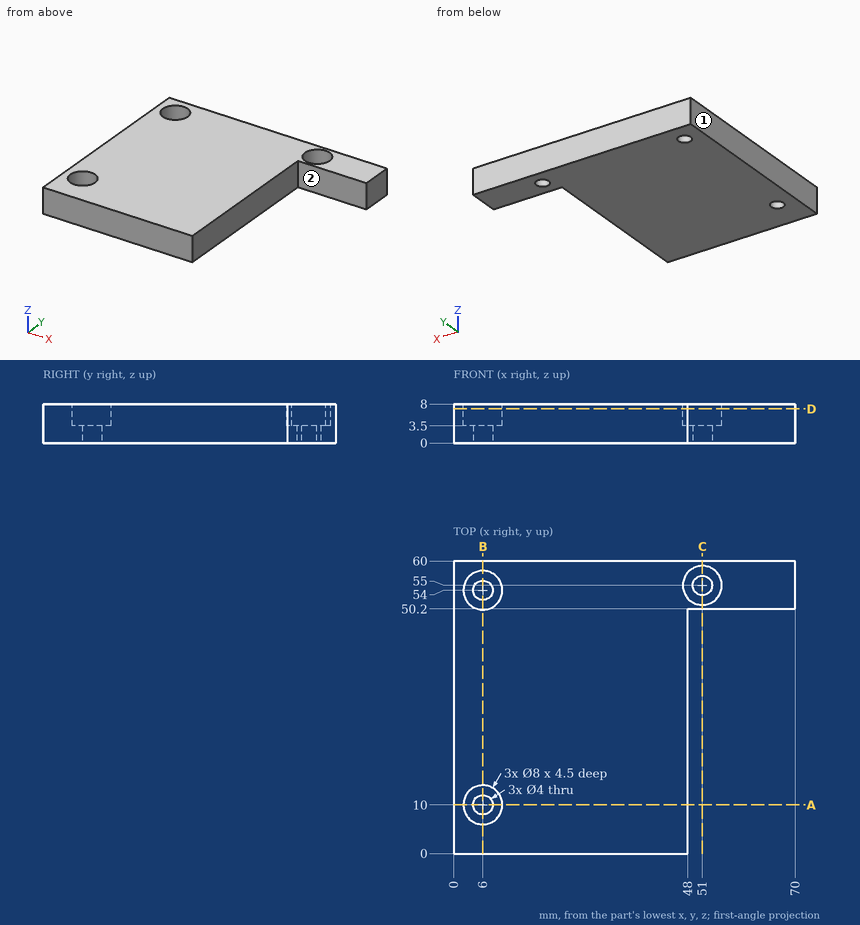
Part print with two shaded views. Sizes in mm from the minimum x, y, z corner. A direction names the side the tool comes from. Round coordinates to 2 decimals unless told otherwise and drop trailing zeros. Order: outer loops, then holes, each group sorted by start corner. A loop starts at its lowest first (then second) coordinate and runs counter-clockwise, first axis right, second up. Notation, with made-up numbers: (25, -27.5) - (29, -27.5) arc R23 cw to (29, 8.5) - close; hole circle Ø3 at (-28.75, 25). An arc over 180 degrees is marked (long way). Return JSON: item names as keys, results as strings.
(1) Wall check: probe 1 along Y at (x, z) = (6, 4.9); probe 2 along Y at (x, z) = (6, 2.5); probe 3 along Y at (x, z) = (59.5, 4.75). Give the ranges that are in metal, low to high. Write a range as from..to.
Answer key:
{"probe 1": "y = 0..6, 14..50, 58..60", "probe 2": "y = 0..8, 12..52, 56..60", "probe 3": "y = 50.2..60"}
(2) Cut at A-A (y = 10). Give the cut face in (x, z), then the cut area to 3 significant figures.
Answer key:
{"outline": "(0, 0) - (4, 0) - (4, 3.5) - (2, 3.5) - (2, 8) - (0, 8) - close; (8, 0) - (48, 0) - (48, 8) - (10, 8) - (10, 3.5) - (8, 3.5) - close", "area": "334 mm^2"}
(3) Cut at D-D (z = 7). Give the cut face in (x, y), then the cut area to 3 significant figures.
Answer key:
{"outline": "(0, 0) - (48, 0) - (48, 50.2) - (70, 50.2) - (70, 60) - (0, 60) - close; hole circle Ø8 at (6, 10); hole circle Ø8 at (6, 54); hole circle Ø8 at (51, 55)", "area": "2,940 mm^2"}
(4) Tool access for the marked faces 1 and 2: list every direction of +Z, -Z, +X, -X, +Y, -Y with a clear straight run to the whole face (end or side of a thin tool).
Answer key:
{"face 1": "+Z, -Z, -X, +Y, -Y", "face 2": "+Z, -Z, +X, -Y"}
(5) Cut at C-C (x = 51). Give the cut face in (y, z).
Answer key:
{"outline": "(50.2, 0) - (53, 0) - (53, 3.5) - (51, 3.5) - (51, 8) - (50.2, 8) - close; (57, 0) - (60, 0) - (60, 8) - (59, 8) - (59, 3.5) - (57, 3.5) - close"}
(6) Pin check, flat tips, straight feed: pin 1 Ø9 at (x, y) = (51, 55) entering from -Z; pin 2 Ø2.5 at (x, y) = (51, 56) entering from +Z; pin 3 Ø2.5 at (x, y) = (6, 54) entering from -Z; pin 4 Ø4 at (y, z) = (19, 3.5) entering from +X. Stop position of each tip, or through.
Answer key:
{"pin 1": "stops at z = 0", "pin 2": "stops at z = 3.5", "pin 3": "passes through", "pin 4": "stops at x = 48"}
(7) Cut at B-B (x = 6). Give the cut face in (y, z).
Answer key:
{"outline": "(0, 0) - (8, 0) - (8, 3.5) - (6, 3.5) - (6, 8) - (0, 8) - close; (12, 0) - (52, 0) - (52, 3.5) - (50, 3.5) - (50, 8) - (14, 8) - (14, 3.5) - (12, 3.5) - close; (56, 0) - (60, 0) - (60, 8) - (58, 8) - (58, 3.5) - (56, 3.5) - close"}
